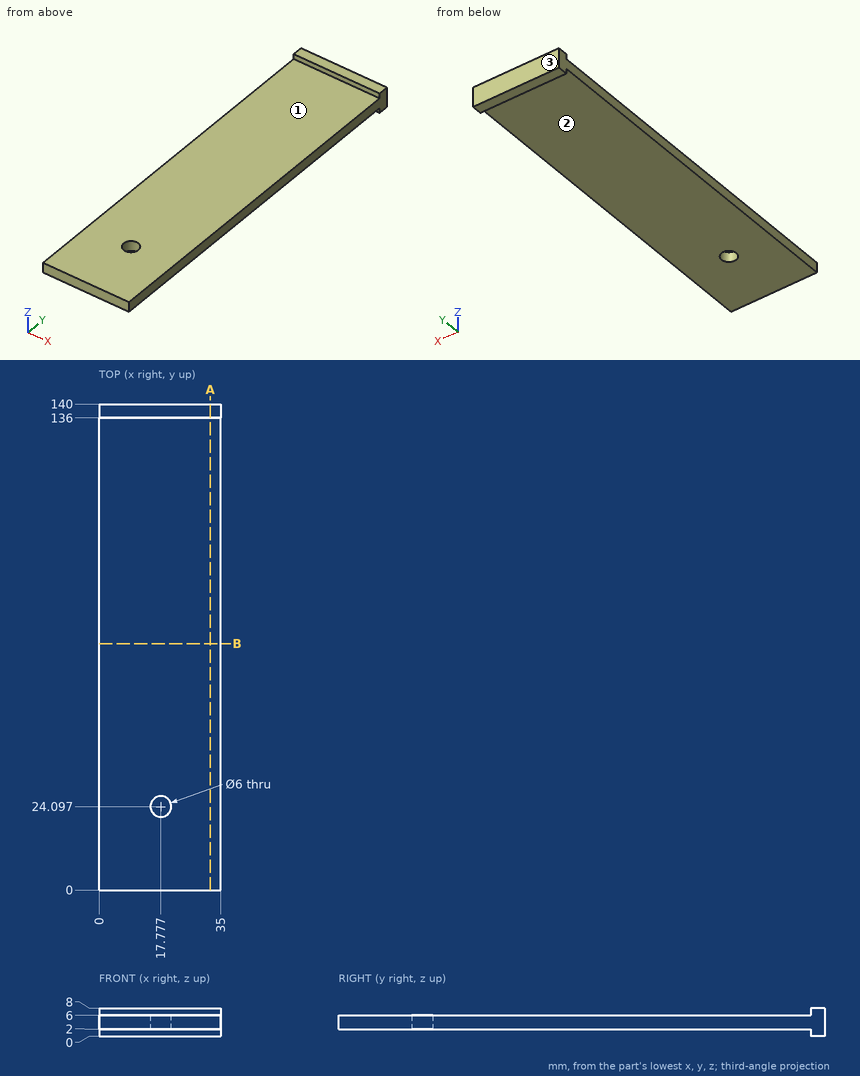
Geometry check sheet. Reference: drawing and pictorial views, mm from the part's lowest x, y, z. A direction names the side the tool comes from. Give positions to 0.01 mm unless a question says otherwise; leave off trailing zeros. Loops run counter-clockwise (first coordinate to the right, second up) from the corner with the lowest first, then second, coordinate; pieces in that order, holes last. Notation, with made-up numbers: (19.5, 45) - (57.5, 45) arc R19 cw to (57.5, 82) - close; hole circle Ø7 at (-36, 7). An arc over 180 degrees is marked (long way). Use CSV: the item, a comma, the result in double quotes. Start each with the question number.
Q1. Go/stop test with flat-tipped pins: pin 1 Ø3 at (x, y) = (4.5, 116.5) entering from +Z; pin 2 Ø1 at (x, z) = (11.5, 1) entering from -Y; pin 3 Ø3 at (x, y) = (14.5, 102) entering from -Z. Record where each tip stops, or that it passes through.
Q2. Section check A-A, the plane x = 32. Record the cut outline in (y, z), and give its area (3 significant figures).
Q3. Section check B-B, the plane y = 71. Record the cut outline in (x, z).
Q4. Access from +Z, -Z, +X, -X, +Y, -Y to the whole of each face (thin tool, end or side, straight path). Record for the marked faces 1, 2 and 3.
Q5. Scan lines: probe 1 along Y at (x, z) = (24.5, 7.75); probe 2 along Z at (x, y) = (15, 44.5); probe 3 along Y at (x, z) = (19, 3) (1 decimal). Record each from-to range of solid material in increasing order. Write a range as from..to.
Findings below:
1,pin 1,"stops at z = 6"
1,pin 2,"stops at y = 136"
1,pin 3,"stops at z = 2"
2,outline,"(0, 2) - (136, 2) - (136, 0) - (140, 0) - (140, 8) - (136, 8) - (136, 6) - (0, 6) - close"
2,area,"576 mm^2"
3,outline,"(0, 2) - (35, 2) - (35, 6) - (0, 6) - close"
4,face 1,"+Z, +X, -X, -Y"
4,face 2,"-Z, +X, -X, -Y"
4,face 3,"+Z, -Z, +X, -X, +Y"
5,probe 1,"y = 136..140"
5,probe 2,"z = 2..6"
5,probe 3,"y = 0..21.4, 26.8..140"
